CAD build for the part. Positions are in the model's coordinates, mm. Face numbers are marked on the shaded views. A direction names the side the tool comes from. Coordinates: 2 decimals unless noted, no trailing zeros. Order: outer loops, then holes, each group sorted by start corner. A loop starts at its lowest first (then second) coordinate and runs counter-clockwise, first axis right, second up. Notation, with made-up numbers: M 24.5,37.5 L 41.5,37.5 A13 ccw 41.5,54.5 Z; hole C 16.5,53 d10. An arc over 180 degrees is marked long. Write item = value, one per line.
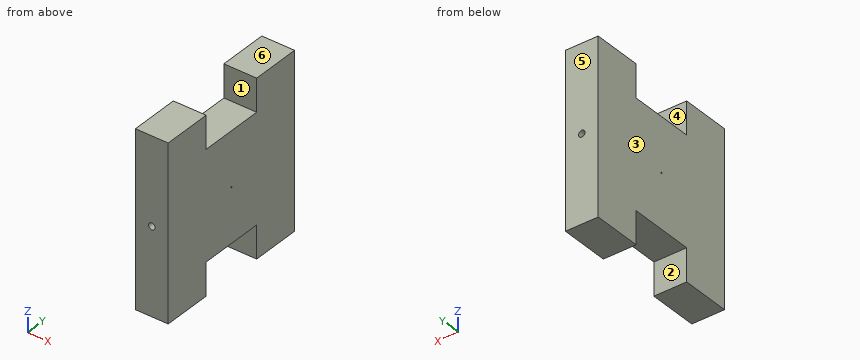
Autodesk Inventor part; units mm, degrees
ref_plane "YZ Plane" through (0, 0, 0) normal (1, 0, 0) x (0, 1, 0)
ref_plane "XZ Plane" through (0, 0, 0) normal (0, 1, 0) x (-1, 0, 0)
ref_plane "XY Plane" through (0, 0, 0) normal (0, 0, 1) x (1, 0, 0)
sketch "Sketch3" plane through (0, 0, 0) normal (1, 0, 0) x (0, 1, 0)
  line L0 (25, -26.5) -> (-25, -26.5)
  line L1 (-25, -26.5) -> (-25, 26.5)
  line L2 (-25, 26.5) -> (25, 26.5)
  line L3 (25, 26.5) -> (25, -26.5)
  line L4 (25, -26.5) -> (-25, 26.5) construction
  line L5 (-25, -26.5) -> (25, 26.5) construction
  line L6 (25, 26.5) -> (10, 26.5)
  line L7 (10, 26.5) -> (10, 16.5)
  line L8 (10, 16.5) -> (-10, 16.5)
  line L9 (-10, 16.5) -> (-10, 26.5)
  line L10 (-10, 26.5) -> (-25, 26.5)
  line L11 (25, -26.5) -> (10, -26.5)
  line L12 (10, -26.5) -> (10, -16.5)
  line L13 (10, -16.5) -> (-10, -16.5)
  line L14 (-10, -16.5) -> (-10, -26.5)
  line L15 (-10, -26.5) -> (-25, -26.5)
  point P0 (0, 0)
  dimension "d0" = 50
  dimension "d1" = 53
  dimension "d2" = 15
  dimension "d3" = 10
  dimension "d4" = 20
  dimension "d5" = 10
  dimension "d6" = 15
  dimension "d7" = 10
  dimension "d8" = 20
  dimension "d9" = 10
  dimension "d10" = 15
extrude "Extrusion1" add sketch "Sketch3" along normal blind 10 contours L0 L12 L13 L14 L1 L2 L9 L8 L7 L3
sketch "Sketch5" plane through (10, 0, 0) normal (1, 0, 0) x (0, 0, -1)
  circle A0 centre (0, 0) radius 0.2
  dimension "d13" = 0.4
hole "Hole1" at (10, 0, 0) direction (-1, 0, 0) diameter 0.4 depth 10
sketch "Sketch6" plane through (0, -25, -26.5) normal (0, -1, 0) x (1, 0, 0)
  circle A0 centre (5, 26.5) radius 2.5
hole "Hole2" at (5, -25, 0) direction (0, 1, 0) diameter 2 depth 50
properties part number "prepazka_kola"
(1) Slice it at D-D, the plane x = 8.75. Write the cut outline in (y, z).
Evaluation:
outline = M -25,-26.5 L -10,-26.5 L -10,-16.5 L 10,-16.5 L 10,-26.5 L 25,-26.5 L 25,26.5 L 10,26.5 L 10,16.5 L -10,16.5 L -10,26.5 L -25,26.5 Z; hole C 0,0 d0.4
(2) Tool access for the marked faces 1, 2 and 3: list every direction of +Z, -Z, +X, -X, +Y, -Y with a clear straight run to the whole face (end or side of a thin tool).
Evaluation:
face_1 = +Z, +X, -X
face_2 = -Z, +X, -X
face_3 = +Z, -Z, -X, +Y, -Y
(3) Pull direction Y, two halves, no side cores. Call the marked faces 4, 5 and 6: +Y half, -Y half, draft (parallel to the pull), parting line (faces both ways), or undercut.
Evaluation:
face_4 = undercut
face_5 = +Y half
face_6 = draft
(4) Wall check: line 1 (Y direction, x = 8.25, z = 18.5); line 2 (Z direction, x = 5, y = 5.5); line 3 (Y direction, x = 2.3, z = 0). Give the ranges that are in metal, low to high. Write a range as from..to.
Evaluation:
line_1 = -25..-10, 10..25
line_2 = -16.5..-1, 1..16.5
line_3 = -25..-0.2, 0.2..25
(5) Slice it at B-B, the plane z = -18.5. Write the cut outline in (x, y).
Evaluation:
outline = M 0,-25 L 10,-25 L 10,-10 L 0,-10 Z; M 0,10 L 10,10 L 10,25 L 0,25 Z
(6) Slice it at C-C, the plane y = 1.5. Write the cut outline in (x, z), then the cut area to 3 significant figures.
Evaluation:
outline = M 0,-16.5 L 10,-16.5 L 10,16.5 L 0,16.5 Z; hole C 5,0 d2
area = 327 mm²
(7) Pin check, flat tips, straight feed: pin 1 Ø2 at (x, y) = (6.5, 3.5) entering from -Z; pin 2 Ø3 at (x, y) = (3.5, 2.5) entering from +Z; pin 3 Ø5 at (y, z) = (19, -20) entering from -X. Stop position of each tip, or through.
Evaluation:
pin_1 = -16.5
pin_2 = 16.5
pin_3 = 0
(8) Slice it at A-A, the plane x = 5. Write the cut outline in (y, z), then the cut area to 3 significant figures.
Evaluation:
outline = M -25,-26.5 L -10,-26.5 L -10,-16.5 L 10,-16.5 L 10,-26.5 L 25,-26.5 L 25,-1 L -25,-1 Z; M -25,1 L 25,1 L 25,26.5 L 10,26.5 L 10,16.5 L -10,16.5 L -10,26.5 L -25,26.5 Z
area = 2,150 mm²
